Input: part model. Units: mm. Frame: model coordinates. A direction names the side the tool comes from. Round coordinates to 2 decimals unless told otherwise and drop trailing zeros. Write each loop counter-clockwise with the first axis right and the second up, starting at its lowest first coordinate (ties: lowest second). Pieces come first, ordered by that corner, then holes. Notation, with made-up numbers: (-32.75, 11) - (-0.75, 11) arc R17 cw to (-0.75, 31) - close; hole circle Ø10 at (0, 40). An arc over 180 degrees is marked (long way). Use one line per item in the form item = value.
```python
from build123d import *

# Parameters (mm, degrees)
SKETCH2_W           = 53.489335428
SKETCH2_H           = 6.35
BOSS_EXTRUDE1_DEPTH = 95.25
SKETCH3_W           = 6.35
SKETCH3_H           = 6.35
CUT_EXTRUDE1_DEPTH  = 7.35
LPATTERN1_COUNT     = 3
LPATTERN1_PITCH     = 19.05
SKETCH5_W           = 15.875
SKETCH5_H           = 6.374255969
SKETCH5_W_2         = 12.7
SKETCH5_H_2         = 6.35
CUT_EXTRUDE2_DEPTH  = 7.35
SKETCH7_W           = 40.64
SKETCH7_H           = 20.32
CUT_EXTRUDE4_DEPTH  = 7.35


with BuildPart() as part:
    # Sketch2 → Boss-Extrude1 (new body)
    with BuildSketch(Plane(origin=(0, 0, 0), x_dir=(0, 0, -1), z_dir=(1, 0, 0))):
        with Locations((30.077985794, 34.925)):
            Rectangle(SKETCH2_W, SKETCH2_H)
    extrude(amount=BOSS_EXTRUDE1_DEPTH)

    # Sketch3 → Cut-Extrude1 (cut, through all)
    with BuildSketch(Plane(origin=(0, 38.1, 0), x_dir=(1, 0, 0), z_dir=(0, 1, 0))):
        with Locations((3.175, 50.472653508)):
            Rectangle(SKETCH3_W, SKETCH3_H)
        with Locations((92.075, 50.472653508)):
            Rectangle(SKETCH3_W, SKETCH3_H)
    cut_extrude1 = extrude(amount=-CUT_EXTRUDE1_DEPTH, mode=Mode.SUBTRACT)

    # LPattern1: Cut-Extrude1 ×3
    with Locations(*[(0, 0, i * LPATTERN1_PITCH) for i in range(1, LPATTERN1_COUNT)]):
        add(cut_extrude1, mode=Mode.SUBTRACT)

    # Sketch5 → Cut-Extrude2 (cut, through all)
    with BuildSketch(Plane(origin=(0, 38.1, 0), x_dir=(1, 0, 0), z_dir=(0, 1, 0))):
        with Locations((7.9375, 6.520446064)):
            Rectangle(SKETCH5_W, SKETCH5_H)
        with Locations((34.925, 6.520446064)):
            Rectangle(SKETCH5_W_2, SKETCH5_H)
        with Locations((60.325, 6.520446064)):
            Rectangle(SKETCH5_W_2, SKETCH5_H)
        with Locations((87.3125, 6.520446064)):
            Rectangle(SKETCH5_W, SKETCH5_H)
        with Locations((7.9375, 53.647653508)):
            Rectangle(SKETCH5_W, SKETCH5_H_2)
        with Locations((34.925, 53.647653508)):
            Rectangle(SKETCH5_W_2, SKETCH5_H_2)
        with Locations((60.325, 53.647653508)):
            Rectangle(SKETCH5_W_2, SKETCH5_H_2)
        with Locations((87.3125, 53.647653508)):
            Rectangle(SKETCH5_W, SKETCH5_H_2)
    extrude(amount=-CUT_EXTRUDE2_DEPTH, mode=Mode.SUBTRACT)

    # Sketch7 → Cut-Extrude4 (cut, through all)
    with BuildSketch(Plane(origin=(0, 38.1, 0), x_dir=(1, 0, 0), z_dir=(0, 1, 0))):
        with Locations((59.85, 37.772653508)):
            Rectangle(SKETCH7_W, SKETCH7_H)
        with BuildLine():
            Line((83.85, 44.522653508), (85.85, 44.522653508))
            ThreePointArc((85.85, 44.522653508), (87.6, 42.772653508), (85.85, 41.022653508))
            Line((85.85, 41.022653508), (83.85, 41.022653508))
            ThreePointArc((83.85, 41.022653508), (82.1, 42.772653508), (83.85, 44.522653508))
        make_face()
        with BuildLine():
            Line((83.85, 34.522653508), (85.85, 34.522653508))
            ThreePointArc((85.85, 34.522653508), (87.6, 32.772653508), (85.85, 31.022653508))
            Line((85.85, 31.022653508), (83.85, 31.022653508))
            ThreePointArc((83.85, 31.022653508), (82.1, 32.772653508), (83.85, 34.522653508))
        make_face()
        with BuildLine():
            Line((35.85, 41.022653508), (33.85, 41.022653508))
            ThreePointArc((33.85, 41.022653508), (32.1, 42.772653508), (33.85, 44.522653508))
            Line((33.85, 44.522653508), (35.85, 44.522653508))
            ThreePointArc((35.85, 44.522653508), (37.6, 42.772653508), (35.85, 41.022653508))
        make_face()
        with BuildLine():
            Line((35.85, 31.022653508), (33.85, 31.022653508))
            ThreePointArc((33.85, 31.022653508), (32.1, 32.772653508), (33.85, 34.522653508))
            Line((33.85, 34.522653508), (35.85, 34.522653508))
            ThreePointArc((35.85, 34.522653508), (37.6, 32.772653508), (35.85, 31.022653508))
        make_face()
    extrude(amount=-CUT_EXTRUDE4_DEPTH, mode=Mode.SUBTRACT)


solid = part.part
```
(1) Draft query along X for faces 1 (the face through (48, 35, -3.333)), 2 (the face through (32.1, 35, -42.7)). Return one class per face: released by +X, released by -X, zero draft, split by the parting line, or undercut.
Derived:
face_1 = zero draft
face_2 = undercut
(2) First-contact query: pin 1 Ø0.6 at (x, y) = (35, 34) entering from -Z; pin 2 Ø1.6 at (x, y) = (85, 36) entering from +Z; pin 3 Ø3 at (y, z) = (36, -13.5) entering from -X. Flat tips, straight axial feed; report the tip coordinate or a pass-through.
Derived:
pin_1 = -50.47
pin_2 = -9.71
pin_3 = 6.35
(3) Access query for faces 3 (the face through (84, 35, -50.473)), 4 (the face through (66.675, 35, -54)), 5 (the face through (92, 35, -34.598)), 6 (the face through (35, 35, -34.523)), 7 (the face through (84, 35, -9.708)). Directions: +Z, -Z, +X, -X, +Y, -Y. A direction counts if a zero-diameter tool reaches every point of the face in a straight line with its end or side. Return the directions, or none.
Derived:
face_3 = -Z, +X, +Y, -Y
face_4 = -Z, +Y, -Y
face_5 = +X, +Y, -Y
face_6 = +Y, -Y
face_7 = +Z, +X, +Y, -Y
(4) Cut plane B-B on z = -12.5. Output: boundary loops of the cut face in (x, y), then the cut area to 3 significant figures.
Derived:
outline = (6.35, 31.75) - (88.9, 31.75) - (88.9, 38.1) - (6.35, 38.1) - close
area = 524 mm^2
(5) Material intervals for L1, parallel to X at y = 33.25, z = -51.5 (3 decimals); L2, parallel to X at y = 36.5, z = -37.5; L3, parallel to Z at x = 47.5, y = 32.25, sorted ascending.
Derived:
L1 = 15.875 to 28.575, 41.275 to 53.975, 66.675 to 79.375
L2 = 0 to 39.53, 80.17 to 95.25
L3 = -56.82 to -47.93, -27.61 to -3.33
(6) Cut plane A-A on z = -7. Output: boundary loops of the cut face in (x, y) (3 decimals).
Derived:
outline = (15.875, 31.75) - (28.575, 31.75) - (28.575, 38.1) - (15.875, 38.1) - close; (41.275, 31.75) - (53.975, 31.75) - (53.975, 38.1) - (41.275, 38.1) - close; (66.675, 31.75) - (79.375, 31.75) - (79.375, 38.1) - (66.675, 38.1) - close
(7) Cut plane C-C on y = 34.5. Count the separate pieces of the cut face and the enclosed holes in it, then the cut area to 3 significant figures.
Derived:
separate_pieces = 1
enclosed_holes = 5
area = 3,280 mm^2
